Verification items for this drawing (mm, ordinates from the low corner). A direction names the side the tool comes from. Coordinates: 2 decimals unless noted, no trailing zeros. Loops run counter-clockwise (first coordinate to the right, second up) from the corner with the lowest first, then second, coordinate; pieces in that order, holes last. Notation, with made-up numbers: M -29,6 L -4,6 A22 cw -4,45 Z; hole C 73.5,71 d10. An arc over 180 degrees is marked long. Return JSON: item names as keys, results as strings.
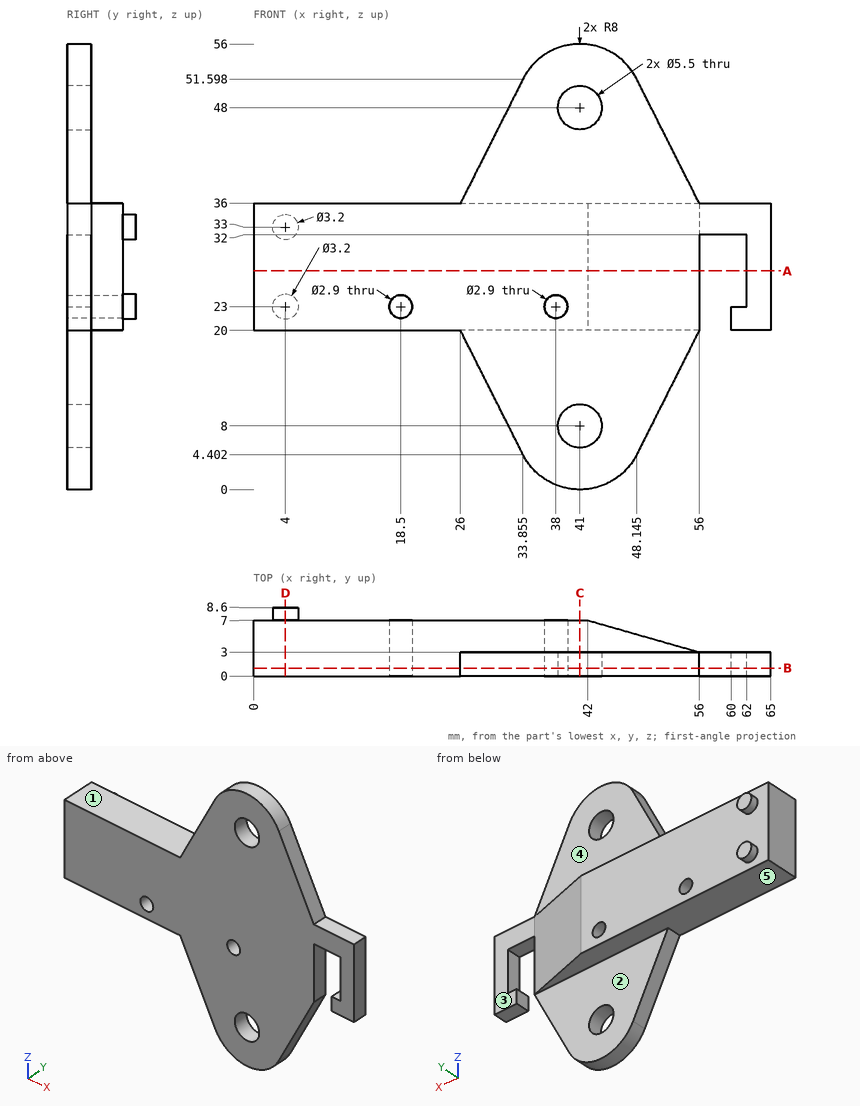
1) Go/stop test with flat-tipped pins: pin 1 Ø3.5 at (x, y) = (63, 2) entering from -Z; pin 2 Ø7 at (x, z) = (58.5, 30.5) entering from +Y; pin 3 Ø6 at (x, z) = (43, 43) entering from +Y. Record where each tip stops, or that it passes through.
Answers:
{"pin 1": "z = 20", "pin 2": "y = 3.29", "pin 3": "y = 3"}
2) Scan lines: line 1 along Z through (x, y) = (18.5, 3.5); line 2 along Y through (x, z) = (33, 7.5); line 3 along Z through (x, y) = (28, 5). Record each from-to range of solid material in increasing order. Write a range as [from, to].
Answers:
{"line 1": "[20, 21.55], [24.45, 36]", "line 2": "[0, 3]", "line 3": "[20, 36]"}
3) Section check D-D on x = 4. Record the cut outline in (y, z).
Answers:
{"outline": "M 0,20 L 7,20 L 7,21.4 L 8.6,21.4 L 8.6,24.6 L 7,24.6 L 7,31.4 L 8.6,31.4 L 8.6,34.6 L 7,34.6 L 7,36 L 0,36 Z"}
4) Section check B-B on y = 1. Count the separate pieces of the cut face and the enclosed holes in it, then the cut area to 3 significant figures.
Answers:
{"separate pieces": "1", "enclosed holes": "4", "area": "1,690 mm²"}
5) Section check C-C on x = 41. Record the cut outline in (y, z), then the cut area to 3 significant figures.
Answers:
{"outline": "M 0,0 L 3,0 L 3,5.25 L 0,5.25 Z; M 0,10.75 L 3,10.75 L 3,20 L 7,20 L 7,36 L 3,36 L 3,45.25 L 0,45.25 Z; M 0,50.75 L 3,50.75 L 3,56 L 0,56 Z", "area": "199 mm²"}
6) Set-up check for the marked faces 1, 2, 3, 4 and 5: record each of +Z, -Z, +X, -X, +Y, -Y from which the full face is reachable in a straight line by a thin tool's end or side.
Answers:
{"face 1": "+Z, -X, +Y", "face 2": "-Z, +X, -X, +Y", "face 3": "+Z, -Z, +X, +Y", "face 4": "+Z, +X, -X, +Y", "face 5": "-Z, -X, +Y"}
7) Section check A-A on z = 27.5. Record the cut outline in (x, y).
Answers:
{"outline": "M 0,0 L 56,0 L 56,3 L 42,7 L 0,7 Z; M 62,0 L 65,0 L 65,3 L 62,3 Z"}
